For this review, take the finished solid that the model builds, in its own axes (mm). A direction names the side the tool comes from. Give positions to 0.01 mm unless a question says otherwise; leave off trailing zeros. Loops run counter-clockwise (first coordinate to the right, second up) from the corner with the lowest first, then second, coordinate; pieces in that order, holes last. Notation, with made-up numbers: (25, -8.75) - (66, -8.75) arc R26 cw to (66, 25.25) - close; hole circle Ø2 at (43.25, 23.25). An arc over 180 degrees is marked (long way). Put each result on its own line as item: value.
from build123d import *

# Parameters (mm, degrees)
SKETCH1_W                          = 80
SKETCH1_H                          = 40
EXTRUDE1_DEPTH                     = 18.9992
F_1_8_0_125_DIAMETER_HOLE1_D       = 3.175
F_1_8_0_125_DIAMETER_HOLE1_DEPTH   = 6.35
F_1_8_0_125_DIAMETER_HOLE1_TIP     = 0.953866233
M3X0_5_TAPPED_HOLE1_D              = 2.5
M3X0_5_TAPPED_HOLE1_DEPTH          = 8.849995
M3X0_5_TAPPED_HOLE1_CBORE_D        = 3
M3X0_5_TAPPED_HOLE1_CBORE_DEPTH    = 6.35
M3X0_5_TAPPED_HOLE1_TIP            = 0.751075774
M5X0_8_TAPPED_HOLE1_D              = 4.2
M5X0_8_TAPPED_HOLE1_CBORE_D        = 5
M5X0_8_TAPPED_HOLE1_CBORE_DEPTH    = 5.08
F_3_16_0_1875_DIAMETER_HOLE1_D     = 4.7625
F_3_16_0_1875_DIAMETER_HOLE1_DEPTH = 6.2484
CUT_REVOLVE1_ANGLE                 = 180
M5X0_8_TAPPED_HOLE2_D              = 4.2
M5X0_8_TAPPED_HOLE2_DEPTH          = 6.6
M5X0_8_TAPPED_HOLE2_CBORE_D        = 5
M5X0_8_TAPPED_HOLE2_CBORE_DEPTH    = 5.08
CIRPATTERN1_COUNT                  = 3
CHAMFER1_SIZE                      = 0.762
EXTRUDE2_DEPTH                     = 0.9906
EXTRUDE3_DEPTH                     = 2.159


with BuildPart() as part:
    # Sketch1 → Extrude1 (new body)
    with BuildSketch(Plane(origin=(0, 0, 0), x_dir=(1, 0, 0), z_dir=(0, 1, 0))):
        Rectangle(SKETCH1_W, SKETCH1_H)
    extrude(amount=EXTRUDE1_DEPTH)

    # 1_8 _0.125_ Diameter Hole1
    with Locations(Plane.XZ):
        with Locations((-20, 0)):
            Hole(F_1_8_0_125_DIAMETER_HOLE1_D / 2, depth=F_1_8_0_125_DIAMETER_HOLE1_DEPTH)
            with Locations((0, 0, -(F_1_8_0_125_DIAMETER_HOLE1_DEPTH + F_1_8_0_125_DIAMETER_HOLE1_TIP / 2))):  # 118° drill point
                Cone(0, F_1_8_0_125_DIAMETER_HOLE1_D / 2, F_1_8_0_125_DIAMETER_HOLE1_TIP, mode=Mode.SUBTRACT)

    # M3x0.5 Tapped Hole1
    with Locations(Plane.XZ):
        with Locations((20, 0)):
            CounterBoreHole(M3X0_5_TAPPED_HOLE1_D / 2, M3X0_5_TAPPED_HOLE1_CBORE_D / 2, M3X0_5_TAPPED_HOLE1_CBORE_DEPTH, depth=M3X0_5_TAPPED_HOLE1_DEPTH)
            with Locations((0, 0, -(M3X0_5_TAPPED_HOLE1_DEPTH + M3X0_5_TAPPED_HOLE1_TIP / 2))):  # 118° drill point
                Cone(0, M3X0_5_TAPPED_HOLE1_D / 2, M3X0_5_TAPPED_HOLE1_TIP, mode=Mode.SUBTRACT)

    # M5x0.8 Tapped Hole1 (through all)
    with Locations(Plane.XZ):
        with Locations((33.4, 0)):
            CounterBoreHole(M5X0_8_TAPPED_HOLE1_D / 2, M5X0_8_TAPPED_HOLE1_CBORE_D / 2, M5X0_8_TAPPED_HOLE1_CBORE_DEPTH)

    # 3_16 _0.1875_ Diameter Hole1
    with Locations(Plane.XZ):
        with Locations((0, 0)):
            Hole(F_3_16_0_1875_DIAMETER_HOLE1_D / 2, depth=F_3_16_0_1875_DIAMETER_HOLE1_DEPTH)

    # Sketch12 → Cut-Revolve1 (revolve, cut)
    with BuildSketch(Plane.XZ.offset(0.508)):
        with BuildLine():
            Line((0, 6.5024), (0, -6.5024))
            ThreePointArc((0, -6.5024), (6.5024, 0), (0, 6.5024))
        make_face()
    revolve(axis=Axis((0, -0.508, 6.5024), (0, 0, 1)), revolution_arc=CUT_REVOLVE1_ANGLE, mode=Mode.SUBTRACT)

    # M5x0.8 Tapped Hole2
    with Locations(Plane(origin=(40, 0, 0), x_dir=(0, 0, -1), z_dir=(1, 0, 0))):
        with Locations((0, 11.5062)):
            CounterBoreHole(M5X0_8_TAPPED_HOLE2_D / 2, M5X0_8_TAPPED_HOLE2_CBORE_D / 2, M5X0_8_TAPPED_HOLE2_CBORE_DEPTH, depth=M5X0_8_TAPPED_HOLE2_DEPTH)

    # Sketch15 → M3x0.5 Tapped Hole2 (revolve, cut)
    with BuildSketch(Plane(origin=(0, 0, -10.795), x_dir=(0, 0, -1), z_dir=(1, 0, 0))):
        Polygon((0, 0), (0, 9.601070774), (1.25, 8.849995), (1.25, 6.35), (1.5, 6.35), (1.5, 0), align=None)
    m3x0_5_tapped_hole2 = revolve(axis=Axis((0, -6.35, -10.795), (0, 1, 0)), mode=Mode.SUBTRACT)

    # CirPattern1: M3x0.5 Tapped Hole2 ×3 about axis
    cirpattern1_axis = Axis((0, 0, 0), (0, 1, 0))
    for i in range(1, CIRPATTERN1_COUNT):
        add(m3x0_5_tapped_hole2.rotate(cirpattern1_axis, i * 360 / CIRPATTERN1_COUNT), mode=Mode.SUBTRACT)

    # Chamfer1
    chamfer1_edges = [part.edges().sort_by_distance(p)[0] for p in [
        (0, 0, -20),
        (40, 0, 0),
        (0, 0, 20),
        (-40, 0, 0),
    ]]
    chamfer(chamfer1_edges, length=CHAMFER1_SIZE)

    # Sketch2 → Extrude2 (add)
    with BuildSketch(Plane(origin=(0, 18.9992, 0), x_dir=(-1, 0, 0), z_dir=(0, 1, 0))):
        with BuildLine():
            Line((35.8725, 19.0475), (-35.8825, 19.0475))
            ThreePointArc((-35.8825, 19.0475), (-38.12756403, 18.11756403), (-39.0575, 15.8725))
            Line((-39.0575, 15.8725), (-39.0575, -15.8775))
            ThreePointArc((-39.0575, -15.8775), (-38.12756403, -18.12256403), (-35.8825, -19.0525))
            Line((-35.8825, -19.0525), (35.8725, -19.0525))
            ThreePointArc((35.8725, -19.0525), (38.11756403, -18.12256403), (39.0475, -15.8775))
            Line((39.0475, -15.8775), (39.0475, 15.8725))
            ThreePointArc((39.0475, 15.8725), (38.11756403, 18.11756403), (35.8725, 19.0475))
        make_face()
    extrude(amount=EXTRUDE2_DEPTH)

    # Sketch17 → Extrude3 (add)
    with BuildSketch(Plane.XZ):
        Polygon((31.0886, -4.003386697), (35.7114, -4.003386697), (38.022930833, 0), (35.7114, 4.003386697), (31.0886, 4.003386697), (28.777069167, 0), align=None)
    extrude(amount=EXTRUDE3_DEPTH)


solid = part.part
1) Take a section at C-C on y = 2.5. State the section outline as (x, z) points (1 decimal).
Geometry check:
outline: (-40, -20) - (40, -20) - (40, 20) - (-40, 20) - close; hole circle Ø3.2 at (-20, 0); hole circle Ø3 at (-9.3, 5.4); hole circle Ø11.5 at (0, 0); hole circle Ø3 at (0, -10.8); hole circle Ø3 at (9.3, 5.4); hole circle Ø3 at (20, 0); hole circle Ø5 at (33.4, 0)
2) For faces 1 (the face through (-38.142, 19.488, 18.093)), 2 (the face through (-38.09, 19.49, -18.15)), 3 (the face through (10.458, 7.582, 4.821)), 4 (the face through (37.496, 12.257, -2.385)), list the 3-axis set-ups (+Z, -Z, +X, -X, +Y, -Y) from which the entire face can be reached by the end or side of a thin tool; tool diameter is ignored.
Geometry check:
face 1: +Z, -X, +Y
face 2: -Z, -X, +Y
face 3: -Y
face 4: +X
3) Take a section at B-B on z = -8. State the section outline as (x, y) points, and give its area (3 significant figures).
Geometry check:
outline: (-40, 0.76) - (-39.24, 0) - (39.24, 0) - (40, 0.76) - (40, 19) - (39.06, 19) - (39.06, 19.99) - (-39.05, 19.99) - (-39.05, 19) - (-40, 19) - close
area: 1,600 mm²
4) Insertion check: pin 1 Ø0.8 at (x, y) = (-16, 19.5) entering from -Z; pin 2 Ø1.1 at (x, y) = (34.5, -1) entering from -Z; pin 3 Ø0.8 at (y, z) = (12, 2) entering from +X. Each pin has a flat end and moves straight along its axis. Give the tip position at first contact, or say it passes through.
Geometry check:
pin 1: stops at z = -19.05
pin 2: stops at z = -4
pin 3: stops at x = 34.92
5) Wall thickness on line 1 (X direction, y = 16.25, z = 0); line 2 (Z direction, x = 20, y = 6.95); line 3 (Z direction, x = 0, y = 3) (3 decimals): over which ranges is each line inside the solid? List them lowest first.
Geometry check:
line 1: x = -40 to 31.3, 35.5 to 40
line 2: z = -20 to -1.25, 1.25 to 20
line 3: z = -20 to -12.295, -9.295 to -5.475, 5.475 to 20
6) Draft analysis for pull direction Z (two halves, no side actions). For faces 5 (the face through (-1, 10, -20)), 6 (the face through (1, 19.99, 0)), 7 (the face through (18.845, 7.617, -0.479)), state which applies: pulls with the +Z half, pulls with the -Z half, needs draft (parallel to the pull), parting line crosses it, or undercut.
Geometry check:
face 5: pulls with the -Z half
face 6: needs draft
face 7: undercut
7) Take a section at A-A on x = -16. State the section outline as (y, z) points, and give its area (3 significant figures).
Geometry check:
outline: (0, -19.24) - (0.76, -20) - (19, -20) - (19, -19.05) - (19.99, -19.05) - (19.99, 19.05) - (19, 19.05) - (19, 20) - (0.76, 20) - (0, 19.24) - close
area: 797 mm²
